Autodesk Inventor part; units mm, degrees
ref_plane "工作平面2" through (0, 11, 0) normal (0, 1, 0) x (-1, 0, 0)
ref_plane "YZ Plane" through (0, 0, 0) normal (1, 0, 0) x (0, 1, 0)
ref_plane "XY Plane" through (0, 0, 0) normal (0, 0, 1) x (1, 0, 0)
sketch "草圖1" plane through (0, 0, 0) normal (0, 1, 0) x (-1, 0, 0)
  circle A0 centre (0, 0) radius 3.15
  circle A1 centre (0, 0) radius 7
  dimension "d0" = 6.3
  dimension "d1" = 14
extrude "擠出1" add sketch "草圖1" along normal blind 100
sketch "草圖2" plane through (0, 100, 0) normal (0, 1, 0) x (1, 0, 0)
  line L0 (0, 0) -> (0, -5) construction
  circle A0 centre (0, 0) radius 7
  line L1 (-4.899, -5) -> (4.899, -5)
  line L2 (0, 0) -> (0, 5) construction
  line L3 (4.899, 5) -> (-4.899, 5)
  point P0 (-5.3619, -4.5)
  point P1 (-5.3619, 4.5)
  point P2 (5.3619, 4.5)
  dimension "d4" = 5
  dimension "d38" = 5
ref_plane "工作平面1" through (0, 50, 0) normal (0, 1, 0) x (-1, 0, 0)
ref_plane "工作平面2" through (0, 11, 0) normal (0, 1, 0) x (-1, 0, 0)
sketch "草圖10" plane through (0, 11, 0) normal (0, 1, 0) x (-1, 0, 0)
  circle A0 centre (0, 0) radius 3.15
  circle A1 centre (0, 0) radius 9.5
  dimension "d30" = 6.3
  dimension "d31" = 19
extrude "擠出9" add sketch "草圖10" against normal blind 3
extrude "擠出11" add sketch "草圖2" along normal blind 10 contours A0 L1 L3
sketch "草圖12" plane through (4.899, 100, -5) normal (0, 0, -1) x (-1, 0, 0)
  circle A0 centre (4.899, 5) radius 1.75
  line L0 (9.798, 0) -> (0, 0)
  arc A1 (11.899, 7.1414) -> (-2.101, 7.1414) centre (4.899, 0) ccw
  line L1 (-2.101, -89) -> (-2.101, 10)
  line L2 (-2.101, 7.1414) -> (-2.101, 0)
  line L3 (-2.101, -89) -> (-2.101, 10)
  line L4 (11.899, -89) -> (11.899, 10)
  line L5 (11.899, 0) -> (-2.101, 0)
  line L6 (11.899, -89) -> (11.899, 10)
  line L7 (11.899, 0) -> (11.899, 7.1414)
  line L8 (11.899, -89) -> (11.899, 10)
  line L9 (-2.101, 7.1414) -> (-2.101, 10)
  line L10 (0, 10) -> (-2.101, 10)
  line L11 (11.899, 10) -> (-2.101, 10)
  line L12 (11.899, 7.1414) -> (11.899, 10)
  point P0 (4.899, -100)
  dimension "d41" = 3.5
  dimension "d44" = 20
extrude "擠出12" cut sketch "草圖12" against normal up to next contours A0
extrude "擠出13" cut sketch "草圖12" against normal up to next contours A1 L11 L4 | L1 L10 L11 A1
sketch "Sketch13" plane through (0, 0, 0) normal (0, -1, 0) x (1, 0, 0)
  circle A0 centre (0, 0) radius 7
  circle A1 centre (0, 0) radius 7
extrude "Extrusion14" cut sketch "Sketch13" against normal blind 1
properties part number "筷子套"
Here's how the part is built. I have some questions about the finished solid (model axes, mm). A direction names the side the tool comes from. Coordinates: 2 decimals unless noted, no trailing zeros. Loops run counter-clockwise (first coordinate to the right, second up) from the corner with the lowest first, then second, coordinate; pieces in that order, holes last.
1. I need wall thicknesses on L1, parallel to Y at x = 0, z = 3; L2, parallel to Z at x = 0, y = 53. Which ranges of each line are inside material? Lowest first, please.
2. Imagine slicing it at A-A, the plane x = -0.5. Please give me the cut outline in (y, z).
3. For P1, Ø5, axis at x = -1, y = 104, coming from the -Z side; P2, Ø4, axis at x = 0, z = 0, coming from the -Y side; P3, Ø3, axis at x = 2.5, z = -3, coming from the +Y side; P4, Ø2, axis at x = 0, y = 105, coming from the -Z side, each with a flat end and sliding along its axis, tell me the tip position at first contact or that it passes through.
4. For faces 5 (the flat face through (4, 11, -6)), 6 (the cylindrical face through (2.5, 49.807, 1.917)), 7 (the flat face through (0, 100, 6)), which set-ups out of +Z, -Z, +X, -X, +Y, -Y let a thin tool reach every point of the face, with its end or its side?
5. Imagine slicing it at C-C, the plane z = 8. Please give me the cut outline in (x, y).
6. Imagine slicing it at B-B, the plane y = 105. Please give me the cut outline in (x, z).
7. If we mould it in two halves opening along Y, with no side actions, what happens to faces 1 (the flat face through (0, 103, -5)), 2 (the flat face through (1.5, 1, -3)), 3 (the cylindrical face through (0.38, 103.29, -0.07)), 4 (the cylindrical face through (0, 110, 0))? For each: pulls with the +Y half, pulls with the -Y half, needs draft (parallel to the pull), parting line crosses it, or undercut.
Taken from the geometry:
1. L1: y = 100 to 103.25, 106.75 to 110
1. L2: z = -7 to -3.15, 3.15 to 7
2. outline: (1, -6.98) - (8, -6.98) - (8, -9.49) - (11, -9.49) - (11, -6.98) - (100, -6.98) - (100, -5) - (103.32, -5) - (103.32, 5) - (100, 5) - (100, 6.98) - (11, 6.98) - (11, 9.49) - (8, 9.49) - (8, 6.98) - (1, 6.98) - (1, 3.11) - (100, 3.11) - (100, -3.11) - (1, -3.11) - close; (106.68, -5) - (109.99, -5) - (109.99, 5) - (106.68, 5) - close
3. P1: stops at z = -5
3. P2: stops at y = 100
3. P3: stops at y = 109.95
3. P4: passes through
4. face 5: +Y
4. face 6: -Y
4. face 7: +Z, +X, -X, +Y
5. outline: (-5.12, 8) - (5.12, 8) - (5.12, 11) - (-5.12, 11) - close
6. outline: (-4.9, -5) - (-1.75, -5) - (-1.75, 5) - (-4.9, 5) arc R7 ccw to start; (1.75, -5) - (4.9, -5) arc R7 ccw to (4.9, 5) - (1.75, 5) - close
7. face 1: needs draft
7. face 2: pulls with the -Y half
7. face 3: undercut
7. face 4: pulls with the +Y half
